Autodesk Fusion 360 part; units mm, degrees
sketch "Sketch1" plane through (0, 0, 0) normal (0, 1, 0) x (1, 0, 0)
  circle A0 centre (0, 0) radius 13
  circle A1 centre (0, 0) radius 7.5
  line L0 (-4.5, 12.1963) -> (-4.5, -6)
  line L1 (4.5, -6) -> (4.5, 12.1963)
  circle A2 centre (0, 0) radius 10 construction
  line L2 (0, 0) -> (7.0711, -7.0711)
  line L3 (0, 0) -> (13, 0) construction
  point P0 (7.0711, -7.0711)
  dimension "d1" = 26
  dimension "d2" = 15
  dimension "d3" = 9
  dimension "d4" = 20
  dimension "d12" = 45
extrude "Extrude1" add sketch "Sketch1" along normal blind 3 contours A0 A1 L0 L1 | A1 L1 L2 | A1 L0 | A1 L1 L2 picked at (8.8444, -6.7794)
hole "Hole1" at (7.0711, 0, 7.0711) direction (0, 1, 0) diameter 4.3 end through all
pattern_circular "C-Pattern1" count 4 over 360 about axis through (0, 1.75, 0) along (0, 1, 0) of "Hole1"
fillet "Fillet1" radius 2 2 edges at (-4.5, 1.5, 6) (4.5, 1.5, 6)
sketch "Sketch2" plane through (0, 3, 0) normal (0, 1, 0) x (-1, 0, 0)
  circle A0 centre (7.0711, 7.0711) radius 2.15
  circle A1 centre (7.0711, -7.0711) radius 2.15
  circle A2 centre (-7.0711, -7.0711) radius 2.15
  circle A3 centre (-7.0711, 7.0711) radius 2.15
  arc A4 (4.5, -12.1963) -> (-4.5, -12.1963) centre (0, 0) ccw
  line L0 (-4.5, -12.1963) -> (-4.5, 4.899)
  arc A5 (-3.4091, 6.6804) -> (-4.5, 4.899) centre (-2.5, 4.899) ccw
  arc A6 (3.4091, 6.6804) -> (-3.4091, 6.6804) centre (0, 0) ccw
  arc A7 (4.5, 4.899) -> (3.4091, 6.6804) centre (2.5, 4.899) ccw
  line L1 (4.5, 4.899) -> (4.5, -12.1963)
Can you work these out from the model? Positions are in its coordinate system, mm. A direction names the side the tool comes from. Coordinates: 2 decimals unless noted, no trailing zeros. Write each loop counter-clockwise with the first axis right and the second up, starting at its lowest first coordinate (ties: lowest second). Pieces come first, ordered by that corner, then holes. Notation, with made-up numbers: M 81,39.25 L 117,39.25 A14 ccw 117,59.25 Z; hole C 74.25,-34 d8. An arc over 180 degrees is marked long. Use one line per item in the form item = value.
Q1. I need wall thicknesses on line 1 along Z through (x, y) = (8, 0.55); line 2 along Z through (x, y) = (5.75, 1.3); line 3 along X through (y, z) = (0.45, 9). Which ranges of each line are inside material? Lowest first, please. Write a range as from..to.
Model answer:
line_1 = -10.25..-9.01, -5.13..5.13, 9.01..10.25
line_2 = -11.66..-8.77, -5.37..5.37, 8.77..11.66
line_3 = -9.38..-8.02, -6.12..6.12, 8.02..9.38
Q2. If we section it at A-A (z = 0): Write out the boundary of the cut face in (x, y), then the cut area to 3 significant figures.
Model answer:
outline = M -13,0 L -4.5,0 L -4.5,3 L -13,3 Z; M 4.5,0 L 13,0 L 13,3 L 4.5,3 Z
area = 51.0 mm^2
Q3. If we section it at C-C (x = 8.75): Write out the boundary of the cut face in (y, z).
Model answer:
outline = M 0,-9.61 L 3,-9.61 L 3,-8.41 L 0,-8.41 Z; M 0,-5.73 L 3,-5.73 L 3,5.73 L 0,5.73 Z; M 0,8.41 L 3,8.41 L 3,9.61 L 0,9.61 Z
Q4. We'd pull the mould along X, two halves only. Please class faces 1 (the flat face through (6, 3, 0)), 2 (the cylindrical face through (0.51, 1.48, 12.99)), 3 (the cylindrical face through (-4.214, 1.521, 5.93)): +X half, -X half, draft (parallel to the pull), parting line (faces both ways), or undercut.
Model answer:
face_1 = draft
face_2 = parting line
face_3 = undercut
Q5. For faces 4 (the cylindrical face through (4.198, 1.521, 5.957)), 5 (the cylindrical face through (-6.43, 1.52, -5.02)), which set-ups out of +Z, -Z, +X, -X, +Y, -Y let a thin tool reach every point of the face, with its end or its side?
Model answer:
face_4 = -Z, +Y, -Y
face_5 = +Y, -Y
Q6. For P1, Ø2.5, axis at x = 7.07, z = -7.07, coming from the -Y side; P2, Ø5, axis at x = -7, z = -3.5, coming from the -Y side; P3, Ø1, axis at y = 1.5, z = 7, coming from the -X side, each with a flat end and sliding along its axis, tell me the tip position at first contact or that it passes through.
Model answer:
P1 = through
P2 = 0
P3 = -11.26
Q7. If we section it at D-D (z = 8): Write out the boundary of the cut face in (x, y).
Model answer:
outline = M -10.25,0 L -9.01,0 L -9.01,3 L -10.25,3 Z; M -5.13,0 L 5.13,0 L 5.13,3 L -5.13,3 Z; M 9.01,0 L 10.25,0 L 10.25,3 L 9.01,3 Z
Q8. If we section it at B-B (y = 0.7): Write out the boundary of the cut face in (x, z), then the cut area to 3 significant figures.
Model answer:
outline = M -4.5,-12.2 L -4.5,4.9 A2 cw -3.41,6.68 A7.5 cw 3.41,6.68 A2 cw 4.5,4.9 L 4.5,-12.2 A13 ccw long Z; hole C -7.07,-7.07 d4.3; hole C -7.07,7.07 d4.3; hole C 7.07,-7.07 d4.3; hole C 7.07,7.07 d4.3
area = 295 mm^2
